Model file for the job. Use its own axes, mm. A direction names the side the tool comes from. Give positions to 0.01 mm unless a question says otherwise; leave off trailing zeros. Loops run counter-clockwise (first coordinate to the right, second up) from the corner with the lowest first, then second, coordinate; pieces in that order, holes last. Notation, with made-up numbers: M 43,-17 L 77,-17 A7 ccw 77,-13 Z; hole C 69,-10 d5. An arc over 180 degrees is marked long. Answer in a Markdown table with one row per item.
```python
from build123d import *

# Parameters (mm, degrees)
F1_DEPTH     = 15
F3_D         = 5.5
F3_DEPTH     = 21
F3_TIP       = 1.6523667023
F5_D         = 5
F6_R         = 4
F7_T1_DEPTH  = 7
F7_T6_ANGLE  = 359.64
F7_T12_ANGLE = 359.64
F7_T18_ANGLE = 359.64
F7_T24_ANGLE = 359.64
F10_DEPTH    = 4.2


# Not quite as in the source:
# - a fillet or chamfer that OpenCascade refuses, or shapes differently, is made with other operations: its cross-section is extruded or revolved along the edge and cut away or added


with BuildPart() as f1:
    # F0 (on Top) → F1 (new body)
    with BuildSketch(Plane.XY):
        Polygon((-17.3867209846, 30), (-22.3867209846, 30), (-22.3867209846, -30), (-17.3867209846, -30), (-17.3867209846, -7.5), (62.6132790154, -7.5), (62.6132790154, 7.5), (-17.3867209846, 7.5), align=None)
    extrude(amount=F1_DEPTH)

    # F3
    with Locations(Plane.YZ.offset(62.6132790154)):
        with Locations((0, 7.5)):
            Hole(F3_D / 2, depth=F3_DEPTH)
            with Locations((0, 0, -(F3_DEPTH + F3_TIP / 2))):  # 118° drill point
                Cone(0, F3_D / 2, F3_TIP, mode=Mode.SUBTRACT)

    # F5 (through all)
    with Locations(Plane.YZ.offset(-17.3867209846)):
        with Locations((-20, 7.5), (20, 7.5)):
            Hole(F5_D / 2)

    # F6
    f6_edges = [f1.edges().sort_by_distance(p)[0] for p in [
        (22.613279, -7.5, 15),
        (22.613279, 7.5, 15),
        (22.613279, -7.5, 0),
        (22.613279, 7.5, 0),
        (-19.886721, -30, 15),
        (-19.886721, -30, 0),
        (-19.886721, 30, 15),
        (-19.886721, 30, 0),
    ]]
    fillet(f6_edges, radius=F6_R)

    # F7: fillet of radius 10 on 2 edges, made by hand

    # F7_s2 → F7_t1 (join)
    with BuildSketch(Plane.XY.offset(4)):
        with BuildLine():
            ThreePointArc((-17.3867209846, -17.5), (-14.4577887965, -10.4289321881), (-7.3867209846, -7.5))
            Line((-7.3867209846, -7.5), (-17.3867209846, -7.5))
            Line((-17.3867209846, -7.5), (-17.3867209846, -17.5))
        make_face()
        with BuildLine():
            ThreePointArc((-17.3867209846, 17.5), (-14.4577887965, 10.4289321881), (-7.3867209846, 7.5))
            Line((-7.3867209846, 7.5), (-17.3867209846, 7.5))
            Line((-17.3867209846, 7.5), (-17.3867209846, 17.5))
        make_face()
    extrude(amount=F7_T1_DEPTH)


with BuildPart() as f7_tool4:
    # F7_s5 → F7_t6 (revolve)
    with BuildSketch(Plane(origin=(0, -0.0249939071, 3.9778515186), x_dir=(1, 0, 0), z_dir=(0, 0.006283144, -0.9999802609))):
        with BuildLine():
            ThreePointArc((-17.3867209846, -17.5250634889), (-14.4577887965, -10.453995677), (-7.3867209846, -7.5250634889))
            Line((-7.3867209846, -7.5250634889), (-17.3867209846, -7.5250634889))
            Line((-17.3867209846, -7.5250634889), (-17.3867209846, -17.5250634889))
        make_face()
    revolve(axis=Axis((-17.3867209846, 3.5, 4), (1, 0, 0)), revolution_arc=F7_T6_ANGLE)

    split(bisect_by=Plane.XY, keep=Keep.TOP)

    split(bisect_by=Plane.XY.offset(15), keep=Keep.BOTTOM)


with BuildPart() as f1_1:
    add(f1.part)

    # F7_t3: union F7_tool4
    add(f7_tool4.part)


with BuildPart() as f7_tool10:
    # F7_s11 → F7_t12 (revolve)
    with BuildSketch(Plane(origin=(0, 0.069251392, 11.0215563129), x_dir=(1, 0, 0), z_dir=(0, 0.006283144, 0.9999802609))):
        with BuildLine():
            ThreePointArc((-17.3867209846, 17.4308163294), (-14.4577887965, 10.3597485175), (-7.3867209846, 7.4308163294))
            Line((-7.3867209846, 7.4308163294), (-17.3867209846, 7.4308163294))
            Line((-17.3867209846, 7.4308163294), (-17.3867209846, 17.4308163294))
        make_face()
    revolve(axis=Axis((-17.3867209846, 3.5, 11), (-1, 0, 0)), revolution_arc=F7_T12_ANGLE)

    split(bisect_by=Plane.XY, keep=Keep.TOP)

    split(bisect_by=Plane.XY.offset(15), keep=Keep.BOTTOM)


with BuildPart() as f1_2:
    add(f1_1.part)

    # F7_t9: union F7_tool10
    add(f7_tool10.part)


with BuildPart() as f7_tool16:
    # F7_s17 → F7_t18 (revolve)
    with BuildSketch(Plane(origin=(0, 0.0249939071, 3.9778515186), x_dir=(1, 0, 0), z_dir=(0, -0.006283144, -0.9999802609))):
        with BuildLine():
            ThreePointArc((-17.3867209846, 17.5250634889), (-14.4577887965, 10.453995677), (-7.3867209846, 7.5250634889))
            Line((-7.3867209846, 7.5250634889), (-17.3867209846, 7.5250634889))
            Line((-17.3867209846, 7.5250634889), (-17.3867209846, 17.5250634889))
        make_face()
    revolve(axis=Axis((-17.3867209846, -3.5, 4), (-1, 0, 0)), revolution_arc=F7_T18_ANGLE)

    split(bisect_by=Plane.XY, keep=Keep.TOP)

    split(bisect_by=Plane.XY.offset(15), keep=Keep.BOTTOM)


with BuildPart() as f1_3:
    add(f1_2.part)

    # F7_t15: union F7_tool16
    add(f7_tool16.part)


with BuildPart() as f7_tool22:
    # F7_s23 → F7_t24 (revolve)
    with BuildSketch(Plane(origin=(0, -0.069251392, 11.0215563129), x_dir=(1, 0, 0), z_dir=(0, -0.006283144, 0.9999802609))):
        with BuildLine():
            ThreePointArc((-17.3867209846, -17.4308163294), (-14.4577887965, -10.3597485175), (-7.3867209846, -7.4308163294))
            Line((-7.3867209846, -7.4308163294), (-17.3867209846, -7.4308163294))
            Line((-17.3867209846, -7.4308163294), (-17.3867209846, -17.4308163294))
        make_face()
    revolve(axis=Axis((-17.3867209846, -3.5, 11), (1, 0, 0)), revolution_arc=F7_T24_ANGLE)

    split(bisect_by=Plane.XY, keep=Keep.TOP)

    split(bisect_by=Plane.XY.offset(15), keep=Keep.BOTTOM)


with BuildPart() as f1_4:
    add(f1_3.part)

    # F7_t21: union F7_tool22
    add(f7_tool22.part)

    # F9 (on offset) → F10 (cut)
    with BuildSketch(Plane.YZ.offset(47.6132790154)):
        Polygon((0, 2.5925227119), (4.25, 5.0462613559), (4.25, 9.9537386441), (4.25, 17.4553611223), (-4.25, 17.4553611223), (-4.25, 9.9537386441), (-4.25, 5.0462613559), align=None)
    extrude(amount=F10_DEPTH, mode=Mode.SUBTRACT)


solid = f1_4.part
```
Q1. Saw through at B-B (x = 23). Give the cut face in (y, z).
Reported:
| item | result |
|---|---|
| outline | M -7.5,4 A4 ccw -3.5,0 L 3.5,0 A4 ccw 7.5,4 L 7.5,11 A4 ccw 3.5,15 L -3.5,15 A4 ccw -7.5,11 Z |
Q2. Probe probe 1 along Y at (x, z) = (44.25, 7.5); probe 2 along Z at (x, y) = (-20.7, 20); probe 3 along Z at (x, y) = (57.5, 0). List the from-to ranges inside material, lowest first.
Reported:
| item | result |
|---|---|
| probe 1 | -7.5 to -2.75, 2.75 to 7.5 |
| probe 2 | 0 to 5, 10 to 15 |
| probe 3 | 0 to 4.75, 10.25 to 15 |
Q3. Saw through at A-A (y = 20). Give the cut face in (x, z), and give its area (3 significant figures).
Reported:
| item | result |
|---|---|
| outline | M -22.39,0 L -17.39,0 L -17.39,5 L -22.39,5 Z; M -22.39,10 L -17.39,10 L -17.39,15 L -22.39,15 Z |
| area | 50.0 mm² |
Q4. 3-axis set-ups, long thin cutter, end or side, ignore diameter. For faces 1 (the face through (57.138, 0.596, 4.815)), 2 (the face through (49.684, 2.095, 3.802)), 3 (the face through (28, 7.5, 7)): which of +Z, -Z, +X, -X, +Y, -Y reach the whole face in a straight line?
Reported:
| item | result |
|---|---|
| face 1 | +X |
| face 2 | +Z |
| face 3 | +Z, -Z, +X, +Y |
Q5. Mould opens along Y. For faces 4 (the face through (-14.54, 10.51, 7.45)), 5 (the face through (28.103, -6.297, 13.859)), 6 (the face through (-20, 22, 6)), 7 (the face through (44.571, 0.596, 4.815)) say: released by +Y, released by -Y, zero draft, split by the parting line, or undercut.
Reported:
| item | result |
|---|---|
| face 4 | released by +Y |
| face 5 | released by -Y |
| face 6 | undercut |
| face 7 | undercut |
Q6. Saw through at C-C (y = -25). Give the cut face in (x, z).
Reported:
| item | result |
|---|---|
| outline | M -22.39,0 L -17.39,0 L -17.39,15 L -22.39,15 Z |
Q7. Drop flat-ended pins along their axis: pin 1 (8 mm diameter, centred on x = 5.5, z = 8, fed in from -Y); pin 2 (7.5 mm diameter, centred on x = 37.5, z = 7.5, fed in from +Y); pin 3 (4 mm diameter, centred on y = -22.5, z = 7, fed in from +X). Give the stop position or say it passes through.
Reported:
| item | result |
|---|---|
| pin 1 | y = -7.5 |
| pin 2 | y = 7.5 |
| pin 3 | x = -17.39 |
